Build history of the part. All positions in model axes, mm. A direction names the side the tool comes from. Give positions to 0.01 mm unless a question says otherwise; leave off trailing zeros. Loops run counter-clockwise (first coordinate to the right, second up) from the corner with the lowest first, then second, coordinate; pieces in that order, holes last. Notation, with made-up numbers: M 60.5,84.5 L 91.5,84.5 A21 ccw 91.5,120.5 Z; hole C 2.5,-31.5 d10. An arc over 180 degrees is marked long. Put each result on its own line as item: value.
Autodesk Inventor part; units mm, degrees
ref_plane "YZ Plane" through (0, 0, 0) normal (1, 0, 0) x (0, 1, 0)
ref_plane "XZ Plane" through (0, 0, 0) normal (0, 1, 0) x (-1, 0, 0)
ref_plane "XY Plane" through (0, 0, 0) normal (0, 0, 1) x (1, 0, 0)
sketch "Sketch1" plane through (0, 0, 0) normal (0, 0, 1) x (1, 0, 0)
  line L0 (0, 0) -> (0, 24)
  line L1 (0, 24) -> (25, 24)
  line L2 (25, 24) -> (25, 20)
  line L3 (25, 20) -> (5, 20)
  line L4 (5, 20) -> (5, 0)
  line L5 (5, 0) -> (0, 0)
  dimension "d0" = 24
  dimension "d1" = 25
  dimension "d2" = 90
  dimension "d3" = 4
  dimension "d4" = 90
  dimension "d5" = 20
extrude "Extrusion1" add sketch "Sketch1" along normal mid plane 20
sketch "Sketch2" plane through (5, 0, 10) normal (1, 0, 0) x (0, 0, -1)
  circle A0 centre (10, 10) radius 2.75
  point P0 (10, 0)
  dimension "d8" = 5.5
extrude "Extrusion2" cut sketch "Sketch2" against normal blind 20
sketch "Sketch3" plane through (0, 24, 10) normal (0, 1, 0) x (1, 0, 0)
  line L0 (0, 20) -> (0, 0)
  line L1 (25, 20) -> (25, 0)
  line L2 (0, 0) -> (25, 0)
  line L3 (25, 0) -> (25, 20)
  line L4 (25, 20) -> (0, 20)
  line L5 (0, 20) -> (0, 0)
  point P0 (0, 10)
extrude "Extrusion3" add sketch "Sketch3" along normal blind 26.5
properties part number "cylinder segment spacer"
Q1. Slice it at A-A (z = 0). List the corners of the cut face in (x, y).
Here are the results:
outline: M 0,0 L 5,0 L 5,7.25 L 0,7.25 Z; M 0,12.75 L 5,12.75 L 5,20 L 25,20 L 25,50.5 L 0,50.5 Z
Q2. Slice it at B-B (y = 10). List the corners of the cut face in (x, z).
Here are the results:
outline: M 0,-10 L 5,-10 L 5,-2.75 L 0,-2.75 Z; M 0,2.75 L 5,2.75 L 5,10 L 0,10 Z
Q3. Mould opens along Z. For faces 1 (the cylindrical face through (2.535, 12.727, 0.358)), 2 (the flat face through (3, 0, 0)), 3 (the flat face through (10, 31, -10)), 4 (the flat face through (10, 31, 10)) say: pulls with the +Z half, pulls with the -Z half, needs draft (parallel to the pull), parting line crosses it, or undercut.
Here are the results:
face 1: undercut
face 2: needs draft
face 3: pulls with the -Z half
face 4: pulls with the +Z half
Q4. Drop flat-ended pins along their axis: pin 1 Ø7 at (y, z) = (10, 0) entering from +X; pin 2 Ø12 at (y, z) = (15, 0.5) entering from -X. Give the stop position or say it passes through.
Here are the results:
pin 1: x = 5
pin 2: x = 0
Q5. Slice it at D-D (y = 19.5). List the corners of the cut face in (x, z).
Here are the results:
outline: M 0,-10 L 5,-10 L 5,10 L 0,10 Z
Q6. Slice it at C-C (x = 3.75). List the corners of the cut face in (y, z).
Here are the results:
outline: M 0,-10 L 50.5,-10 L 50.5,10 L 0,10 Z; hole C 10,0 d5.5
Q7. Tool access for faces 5 (the flat face through (15, 20, 0)), 6 (the flat face through (12, 50.5, 0)): list every direction of +Z, -Z, +X, -X, +Y, -Y with a clear straight run to the whole face (end or side of a thin tool).
Here are the results:
face 5: +Z, -Z, +X, -Y
face 6: +Z, -Z, +X, -X, +Y
Q8. Probe line 1 (Y direction, x = 1.45, z = 0); line 2 (Y direction, x = 6.25, z = 5); line 3 (X direction, y = 3, z = -8.75). List the from-to ranges inside material, lowest first. Write a range as from..to.
Here are the results:
line 1: 0..7.25, 12.75..50.5
line 2: 20..50.5
line 3: 0..5
